Source: three-view drawing plus pictorial views. Frame: mm from the lowest corner of the part. Give positions to 0.01 mm unless a question says otherwise; leave off trailing zeros. Loops run counter-clockwise (first coordinate to the right, second up) from the corner with the lowest first, then second, coordinate; pieces in that order, holes last. Notation, with made-up numbers: (-38, 68.5) - (5, 68.5) arc R26 cw to (5, 83.5) - close; hole circle Ø2 at (-10.5, 49). An arc over 180 degrees is marked (long way). One line per item, written item: value.
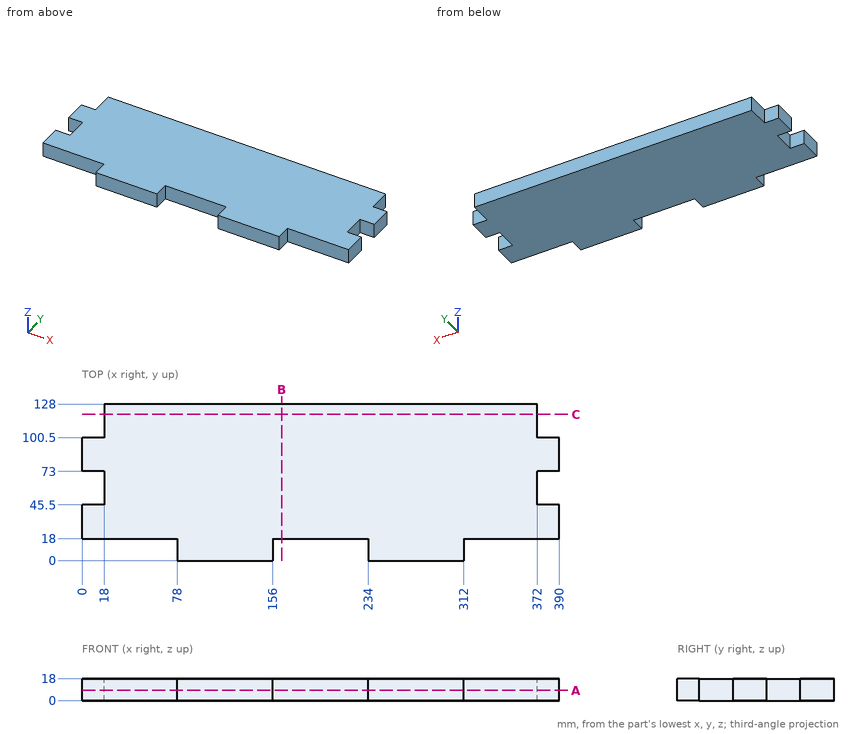
Item 1: Section C-C, the plane y = 119.5. Output: boundary loops of the cut face in (x, z), and give its area (3 significant figures).
Verdict:
outline: (18, 0) - (372, 0) - (372, 18) - (18, 18) - close
area: 6,370 mm^2
Item 2: Material intervals for L1, parallel to X at y = 17.5, z = 13.5; L2, parallel to X at y = 51.5, z = 4.25; L3, parallel to Y at x = 156.5, z = 8.5, sorted ascending.
Verdict:
L1: x = 78 to 156, 234 to 312
L2: x = 18 to 372
L3: y = 18 to 128
Item 3: Pin query (flat end, axial travel): P1, Ø1.5, axis at y = 53, z = 9, coming from the -X side; P2, Ø9, axis at y = 5.5, z = 12, coming from the +X side; P3, Ø9, axis at x = 379.5, z = 11.5, coming from the -Y side. Return the tip coordinate at first contact, or that it passes through.
Verdict:
P1: stops at x = 18
P2: stops at x = 312
P3: stops at y = 18
Item 4: Section A-A, the plane z = 8.5. Output: boundary loops of the cut face in (x, y), and give its area (3 significant figures).
Verdict:
outline: (0, 18) - (78, 18) - (78, 0) - (156, 0) - (156, 18) - (234, 18) - (234, 0) - (312, 0) - (312, 18) - (390, 18) - (390, 45.5) - (372, 45.5) - (372, 73) - (390, 73) - (390, 100.5) - (372, 100.5) - (372, 128) - (18, 128) - (18, 100.5) - (0, 100.5) - (0, 73) - (18, 73) - (18, 45.5) - (0, 45.5) - close
area: 43,700 mm^2
Item 5: Section B-B, the plane x = 163. Output: boundary loops of the cut face in (y, z).
Verdict:
outline: (18, 0) - (128, 0) - (128, 18) - (18, 18) - close
